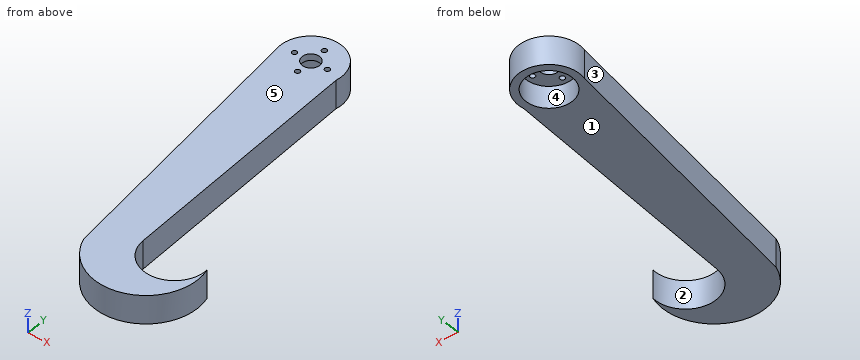
```python
from build123d import *

# Parameters (mm, degrees)
SKETCH_1_R          = 14
EXTRUDE_1_DEPTH     = 13
SKETCH_2_R          = 10.6
CUT_EXTRUDE_1_DEPTH = 10
SKETCH_3_R          = 4
CUT_EXTRUDE_2_DEPTH = 10
EXTRUDE_START       = -13
EXTRUDE_3_DEPTH     = 13
SKETCH_7_R          = 1.15
CUT_EXTRUDE_3_DEPTH = 14


with BuildPart() as part:
    # 스케치1 → 보스-돌출1 (new body)
    with BuildSketch(Plane.XY):
        with Locations(Location((0, 0, 0), (0, 0, 180))):
            Circle(SKETCH_1_R)
    extrude(amount=EXTRUDE_1_DEPTH)

    # 스케치2 → 컷-돌출1 (cut)
    with BuildSketch(Plane(origin=(0, 0, 0), x_dir=(-1, 0, 0), z_dir=(0, 0, -1))):
        Circle(SKETCH_2_R)
    extrude(amount=-CUT_EXTRUDE_1_DEPTH, mode=Mode.SUBTRACT)

    # 스케치3 → 컷-돌출2 (cut)
    with BuildSketch(Plane.XY.offset(13)):
        Circle(SKETCH_3_R)
    extrude(amount=-CUT_EXTRUDE_2_DEPTH, mode=Mode.SUBTRACT)

    # 스케치6 → 보스-돌출3 (add)
    with BuildSketch(Plane.XY.offset(13).offset(EXTRUDE_START)):
        with BuildLine():
            Line((13.735578357, -2.708115061), (17.539668143, -115.708115061))
            ThreePointArc((17.539668143, -115.708115061), (32.332669837, -129.214149758), (45.486033392, -114.10670459))
            ThreePointArc((45.486033392, -114.10670459), (29.938586036, -143.187708961), (0.608578272, -128.115264599))
            Line((0.608578272, -128.115264599), (-13.64899727, -3.115264599))
            ThreePointArc((-13.64899727, -3.115264599), (0.208126783, -13.998452887), (13.735578357, -2.708115061))
        make_face()
    extrude(amount=EXTRUDE_3_DEPTH)

    # 스케치7 → 컷-돌출3 (cut)
    with BuildSketch(Plane(origin=(0, 0, 10), x_dir=(-1, 0, 0), z_dir=(0, 0, -1))):
        with Locations((7.5, 0)):
            Circle(SKETCH_7_R)
        with Locations((0, -7.5)):
            Circle(SKETCH_7_R)
        with Locations((-7.5, 0)):
            Circle(SKETCH_7_R)
        with Locations((0, 7.5)):
            Circle(SKETCH_7_R)
    extrude(amount=-CUT_EXTRUDE_3_DEPTH, mode=Mode.SUBTRACT)


solid = part.part
```
Check sheet for the modelled part. Datum: model origin and axes. Units: mm. Face numbers are marked on the shaded views. A direction names the side the tool comes from. Round coordinates to 2 decimals unless told otherwise and drop trailing zeros. Order: outer loops, then holes, each group sorted by start corner. A loop starts at its lowest first (then second) coordinate and runs counter-clockwise, first axis right, second up. Notation, with made-up numbers: (-1.5, -29) - (5.5, -29) arc R23 cw to (5.5, 8) - close; hole circle Ø3 at (-39, -25). An arc over 180 degrees is marked (long way). Write item = value, one per line.
Q1. Thickness scan on line 1 along Y through (x, z) = (4.5, 6); line 2 along X through (y, z) = (-122.5, 8.5); line 3 along Y through (x, z) = (7.5, 11.85). Record the ranges inside material, lowest first.
Computed:
line_1 = -135.34 to -9.6, 9.6 to 13.26
line_2 = -0.03 to 19.56, 43.5 to 46.38
line_3 = -138.48 to -1.15, 1.15 to 11.82
Q2. Tool access check on the marked faces 4 and 5. Record the directions out of +Z, -Z, +X, -X, +Y, -Y that give a thin tool (end or side, any length) a straight path to the whole face; none if there is none.
Computed:
face_4 = -Z
face_5 = +Z, +X, -X, +Y, -Y
Q3. Section check B-B (z = 1.5). Record the boundary of the cut face in (x, y), and give its area (3 significant figures).
Computed:
outline = (-13.65, -3.12) - (0.61, -128.12) arc R23.51 ccw to (45.49, -114.11) arc R14 cw (long way) to (17.54, -115.71) - (13.74, -2.71) arc R14 ccw (long way) to start; hole circle Ø21.2 at (0, 0)
area = 3,420 mm^2
Q4. Draft check along X on the marked faces 1, 2 and 3. Enter one of: pulls with the +X half, pulls with the -X half, needs draft (parallel to the pull), parting line crosses it, or undercut.
Computed:
face_1 = needs draft
face_2 = undercut
face_3 = pulls with the -X half
Q5. Section check A-A (z = 11.5). Record the boundary of the cut face in (x, y), and give its area (3 significant figures).
Computed:
outline = (-13.65, -3.12) - (0.61, -128.12) arc R23.51 ccw to (45.49, -114.11) arc R14 cw (long way) to (17.54, -115.71) - (13.74, -2.71) arc R14 ccw (long way) to start; hole circle Ø2.3 at (-7.5, 0); hole circle Ø8 at (0, 0); hole circle Ø2.3 at (0, -7.5); hole circle Ø2.3 at (0, 7.5); hole circle Ø2.3 at (7.5, 0)
area = 3,710 mm^2
Q6. Go/stop test with flat-tipped pins: pin 1 (1.8 mm diameter, centred on x = -7.5, y = 0, fed in from +Z); pin 2 (1.5 mm diameter, centred on y = -91, z = 10, fed in from +X); pin 3 (2.5 mm diameter, centred on x = 0, y = -7.5, fed in from -Z); pin 4 (2 mm diameter, centred on y = -90, z = 6, fed in from -X). Record where each tip stops, or that it passes through.
Computed:
pin_1 = through
pin_2 = 16.73
pin_3 = 10
pin_4 = -3.85
Q7. Section check C-C (x = 32). Record the boundary of the cut face in (y, z).
Computed:
outline = (-142.44, 0) - (-129.23, 0) - (-129.23, 13) - (-142.44, 13) - close
Q8. Section check D-D (y = -77). Record the boundary of the cut face in (x, z), and give its area (3 significant figures).
Computed:
outline = (-5.22, 0) - (16.24, 0) - (16.24, 13) - (-5.22, 13) - close
area = 279 mm^2
